Read the model definition and answer for the solid it produces. Units are mm, in the model's axes. Face numbers are marked on the shaded views. A direction names the side the tool comes from. Coordinates: 2 decimals unless noted, no trailing zeros. Loops run counter-clockwise (first coordinate to the right, second up) from the corner with the lowest first, then second, coordinate; pieces in that order, holes last. Notation, with made-up numbers: (71, 79) - (75, 79) arc R24 ccw to (75, 91) - close; hole circle Ø9 at (54, 9.25). An arc over 180 degrees is marked (long way). Use CSV: the item, a comma, the result in double quotes.
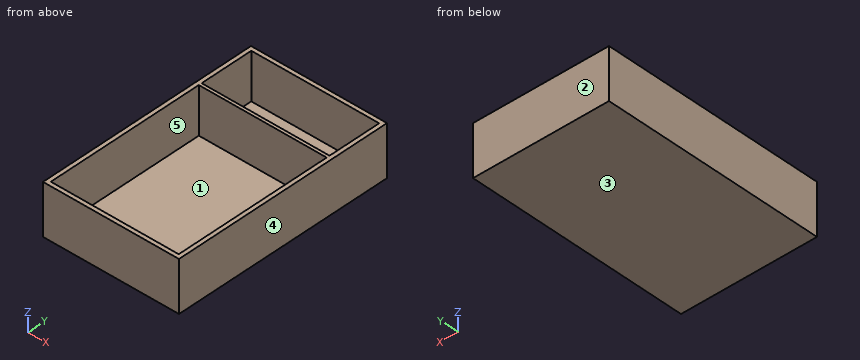
```python
from build123d import *

# Parameters (mm, degrees)
SKETCH022_W    = 67
SKETCH022_H    = 110
PAD009_DEPTH   = 25
THICKNESS002_T = -2
SKETCH023_W    = 1.5
SKETCH023_H    = 25
PAD010_DEPTH   = 63


with BuildPart() as part:
    # Sketch022 → Pad009 (new body)
    with BuildSketch(Plane.XY):
        Rectangle(SKETCH022_W, SKETCH022_H)
    extrude(amount=PAD009_DEPTH)

    # Thickness002
    thickness002_openings = [part.faces().sort_by_distance(p)[0] for p in [
        (0, 0, 25),
    ]]
    offset(amount=THICKNESS002_T, openings=thickness002_openings)

    # Sketch023 (on DatumPlane) → Pad010 (join)
    with BuildSketch(Plane(origin=(-31.5, 26, 0), x_dir=(0, 1, 0), z_dir=(1, 0, 0))):
        with Locations((0, 12.5)):
            Rectangle(SKETCH023_W, SKETCH023_H)
    extrude(amount=PAD010_DEPTH)


with BuildPart() as part_1:
    # Body010 placement: moved
    add(part.part.moved(Location((-61, -60, 0))))


solid = part_1.part
```
Q1. Find the intervals of material crossed by probe 1 along Y at (x, z) = (-55, 17.25); probe 2 along X at (y, z) = (-105.5, 11.25); probe 3 along Z at (x, y) = (-64.5, -44.5), in increasing order. Write a range as [from, to].
Reported:
probe 1,"y = [-115, -113], [-34.75, -33.25], [-7, -5]"
probe 2,"x = [-94.5, -92.5], [-29.5, -27.5]"
probe 3,"z = [0, 2]"
Q2. For a pull along X with two mould halves and no side action, classify the marked faces 3, 4 and 5 as +X half, -X half, draft (parallel to the pull), parting line (faces both ways), or undercut.
Reported:
face 3,"draft"
face 4,"+X half"
face 5,"undercut"
Q3. A tool of negligible diameter and unlimited length cuts with its end or side. For the marked faces 1 and 2, from which of +Z, -Z, +X, -X, +Y, -Y can it reach the whole face along a straight path? Write none if from no direction.
Reported:
face 1,"+Z"
face 2,"+Z, -Z, +X, -X, +Y"
Q4. The part is cut by section B-B on x = -64. Determine the outline of the cut face in (y, z).
Reported:
outline,"(-115, 0) - (-5, 0) - (-5, 25) - (-7, 25) - (-7, 2) - (-33.25, 2) - (-33.25, 25) - (-34.75, 25) - (-34.75, 2) - (-113, 2) - (-113, 25) - (-115, 25) - close"
Q5. The part is cut by section C-C on y = -75. Determine the outline of the cut face in (x, z).
Reported:
outline,"(-94.5, 0) - (-27.5, 0) - (-27.5, 25) - (-29.5, 25) - (-29.5, 2) - (-92.5, 2) - (-92.5, 25) - (-94.5, 25) - close"
Q6. The part is cut by section A-A on z = 7.25. Determine the outline of the cut face in (x, y), and give its area (4 significant figures).
Reported:
outline,"(-94.5, -115) - (-27.5, -115) - (-27.5, -5) - (-94.5, -5) - close; hole (-92.5, -113) - (-29.5, -113) - (-29.5, -34.75) - (-92.5, -34.75) - close; hole (-92.5, -33.25) - (-29.5, -33.25) - (-29.5, -7) - (-92.5, -7) - close"
area,"786.5 mm²"
Q7. Given P1, Ø1, axis at x = -74.5, y = -47, coming from the +Z side, flat-ended and moving along its own axis, determine where the tip first touches the part or whether it passes through.
Reported:
P1,"stops at z = 2"
